from build123d import *

# Parameters (mm, degrees)
BOSS_EXTRUDE1_DEPTH = 20


with BuildPart() as part:
    # Sketch3 → Boss-Extrude1 (new body)
    with BuildSketch(Plane.XY):
        with BuildLine():
            Line((3.750000228, -10), (8.5, -10))
            Line((8.5, -10), (8.5, -11))
            Line((8.5, -11), (-8.5, -11))
            Line((-8.5, -11), (-8.5, -10))
            Line((-8.5, -10), (-3.750000228, -10))
            ThreePointArc((-3.750000228, -10), (-3.608578871, -9.941421356), (-3.550000228, -9.8))
            Line((-3.550000228, -9.8), (-3.550000228, -9.7))
            ThreePointArc((-3.550000228, -9.7), (-3.491421584, -9.558578644), (-3.350000228, -9.5))
            Line((-3.350000228, -9.5), (-3.2, -9.5))
            ThreePointArc((-3.2, -9.5), (-3.058578644, -9.441421356), (-3, -9.3))
            Line((-3, -9.3), (-3, -8.999999673))
            ThreePointArc((-3, -8.999999673), (-3.146446609, -8.646446283), (-3.5, -8.499999673))
            Line((-3.5, -8.499999673), (-5.500000686, -8.499999673))
            ThreePointArc((-5.500000686, -8.499999673), (-5.853554077, -8.353553064), (-6.000000686, -7.999999673))
            Line((-6.000000686, -7.999999673), (-6.000000686, -7.267766626))
            ThreePointArc((-6.000000686, -7.267766626), (-5.961940448, -7.076424899), (-5.853554059, -6.914213219))
            Line((-5.853554059, -6.914213219), (-3.585787212, -4.646446592))
            ThreePointArc((-3.585787212, -4.646446592), (-3.423575544, -4.538060229), (-3.232233839, -4.5))
            Line((-3.232233839, -4.5), (-0.953590312, -4.5))
            ThreePointArc((-0.953590312, -4.5), (-0.901826505, -4.493185166), (-0.853590316, -4.473205083))
            Line((-0.853590316, -4.473205083), (-0.100000045, -4.038119562))
            ThreePointArc((-0.100000045, -4.038119562), (0, -4.011324632), (0.100000045, -4.038119562))
            Line((0.100000045, -4.038119562), (0.853590316, -4.473205083))
            ThreePointArc((0.853590316, -4.473205083), (0.901826505, -4.493185166), (0.953590312, -4.5))
            Line((0.953590312, -4.5), (3.232233839, -4.5))
            ThreePointArc((3.232233839, -4.5), (3.423575544, -4.538060229), (3.585787212, -4.646446592))
            Line((3.585787212, -4.646446592), (5.853554059, -6.914213219))
            ThreePointArc((5.853554059, -6.914213219), (5.961940448, -7.076424899), (6.000000686, -7.267766626))
            Line((6.000000686, -7.267766626), (6.000000686, -7.999999673))
            ThreePointArc((6.000000686, -7.999999673), (5.853554077, -8.353553064), (5.500000686, -8.499999673))
            Line((5.500000686, -8.499999673), (3.5, -8.499999673))
            ThreePointArc((3.5, -8.499999673), (3.146446609, -8.646446283), (3, -8.999999673))
            Line((3, -8.999999673), (3, -9.3))
            ThreePointArc((3, -9.3), (3.058578644, -9.441421356), (3.2, -9.5))
            Line((3.2, -9.5), (3.350000228, -9.5))
            ThreePointArc((3.350000228, -9.5), (3.491421584, -9.558578644), (3.550000228, -9.7))
            Line((3.550000228, -9.7), (3.550000228, -9.8))
            ThreePointArc((3.550000228, -9.8), (3.608578871, -9.941421356), (3.750000228, -10))
        make_face()
    extrude(amount=BOSS_EXTRUDE1_DEPTH)

    # Çizim2 → section 0 of loft1
    with BuildSketch(Plane(origin=(0, -21, 0), x_dir=(-1, 0, 0), z_dir=(0, -1, 0)), mode=Mode.PRIVATE) as loft1_s0:
        with BuildLine():
            Line((-0.560549313, -9.5), (0.439450687, -9.5))
            Line((0.439450687, -9.5), (0.439450687, -10.5))
            Line((0.439450687, -10.5), (-0.560549313, -10.5))
            Line((-0.560549313, -10.5), (-0.560549313, -9.5))
        make_face()
    # loft up to a face of the part (loft1)
    loft([loft1_s0.sketch, part.faces().sort_by_distance((0, -11, 10))[0]])


solid = part.part
Design review of the part built by this model. Coordinates are the model's own, in mm. A direction names the side the tool comes from. Give positions to 0.01 mm unless a question says otherwise; leave off trailing zeros.
1. Tool access review of faces 4 (the flat face through (-6, -10, 10)), 5 (the flat face through (2, -4.5, 10)), 6 (the flat face through (5, -8.5, 10)), 7 (the flat face through (-2, -4.5, 10)): name each direction out of +Z, -Z, +X, -X, +Y, -Y from which nothing blocks a thin tool from reaching the whole face with its end or side.
Solution:
face 4: +Z, -Z, -X
face 5: +Z, -Z, +X, +Y
face 6: +Z, -Z, +X
face 7: +Z, -Z, -X, +Y
2. Mouldability with a two-part tool opening along Y and no side actions: class faces 1 (the flat face through (-8.5, -10.5, 9.9)), 2 (the flat face through (4.7, -5.76, 9.86)), 3 (the flat face through (6, -10, 10)) as +Y half, -Y half, draft (parallel to the pull), parting line (faces both ways), or undercut.
Solution:
face 1: draft
face 2: +Y half
face 3: undercut
3. To check wall thickness, follow L1, parallel to Y at x = -5, z = 13.5; L2, parallel to Y at x = 4.75, z = 6.75; L3, parallel to X at y = -16.75, z = 8.25. State the ranges of each line that lie inside material, in increasing order.
Solution:
L1: y = -15.34 to -10, -8.5 to -6.06
L2: y = -15.72 to -10, -8.5 to -5.81
L3: x = -3.87 to 3.93
4. For pin 1 Ø6 at (y, z) = (-16, 14.5) entering from +X; pin 2 Ø3 at (x, y) = (2, -15) entering from +Z (3 decimals); pin 3 Ø0.7 at (x, z) = (-2, 12.5) entering from +Y, all flat-tipped, find the tip position at first contact; note any pin that passes through.
Solution:
pin 1: stops at x = 6.91
pin 2: stops at z = 17.625
pin 3: stops at y = -4.5
